The listing builds one solid part. Answer for the finished solid, in the listing's coordinates (mm). Face numbers are marked on the shaded views. A direction names the side the tool comes from. Coordinates: 2 decimals unless noted, no trailing zeros. Loops run counter-clockwise (first coordinate to the right, second up) from the corner with the lowest first, then second, coordinate; pieces in that order, holes last. Notation, with made-up numbers: (7, 74.5) - (15, 74.5) arc R23 ccw to (15, 103.5) - close; hole circle Ø8 at (32, 31.25). An arc over 180 degrees is marked (long way). Put each result on its own line as item: value.
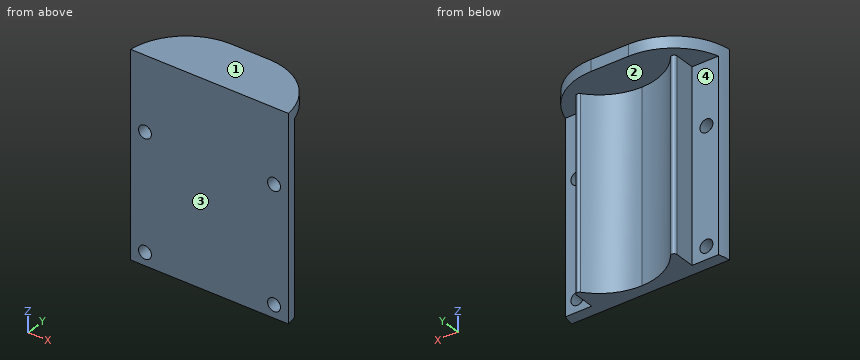
```python
from build123d import *

# Parameters (mm, degrees)
SKETCH1_W            = 55
SKETCH1_H            = 70
BOSS_EXTRUDE1_DEPTH  = 4
M4_CLEARANCE_HOLE1_D = 4.5
BOSS_EXTRUDE2_DEPTH  = 70
SKETCH5_W            = 55
SKETCH5_H            = 4
BOSS_EXTRUDE3_DEPTH  = 15
FILLET1_R            = 1
FILLET2_START        = -36
FILLET2_DEPTH        = 71


with BuildPart() as part:
    # Sketch1 → Boss-Extrude1 (new body)
    with BuildSketch(Plane(origin=(0, 0, 0), x_dir=(1, 0, 0), z_dir=(0, 1, 0))):
        Rectangle(SKETCH1_W, SKETCH1_H)
    extrude(amount=BOSS_EXTRUDE1_DEPTH)

    # M4 Clearance Hole1 (through all)
    with Locations(Plane(origin=(0, 4, 0), x_dir=(1, 0, 0), z_dir=(0, 1, 0))):
        with Locations((-22.5, 30.536735359), (22.5, 30.536735359), (-22.5, -9.463264641), (22.5, -9.463264641)):
            Hole(M4_CLEARANCE_HOLE1_D / 2)

    # Sketch4 → Boss-Extrude2 (add, through all)
    with BuildSketch(Plane(origin=(0, 0, -35), x_dir=(-1, 0, 0), z_dir=(0, 0, -1))):
        with BuildLine():
            Line((-17.5, 14.317541634), (-17.5, 4))
            Line((-17.5, 4), (0, 4))
            ThreePointArc((0, 4), (-10.157530032, 6.771402156), (-17.5, 14.317541634))
        make_face()
        with BuildLine():
            ThreePointArc((17.5, 14.317541634), (10.157530032, 6.771402156), (0, 4))
            Line((0, 4), (17.5, 4))
            Line((17.5, 4), (17.5, 14.317541634))
        make_face()
    extrude(amount=-BOSS_EXTRUDE2_DEPTH)

    # Sketch5 → Boss-Extrude3 (add)
    with BuildSketch(Plane(origin=(0, 4, 0), x_dir=(1, 0, 0), z_dir=(0, 1, 0))):
        with Locations((0, -33)):
            Rectangle(SKETCH5_W, SKETCH5_H)
    extrude(amount=BOSS_EXTRUDE3_DEPTH)

    # Fillet1
    fillet1_edges = [part.edges().sort_by_distance(p)[0] for p in [
        (-17.5, 14.317541634, -2),
        (17.5, 14.317541634, -2),
    ]]
    fillet(fillet1_edges, radius=FILLET1_R)

    # Fillet2: read off the stored shape, not the designer's step
    # Fillet2 outline → Fillet2 (cut)
    with BuildSketch(Plane.XY.offset(FILLET2_START)):
        with BuildLine():
            ThreePointArc((-27.5, 0), (-20.719901931, 13.540270268), (-6.59545504, 19))
            Line((-6.59545504, 19), (-27.5, 19))
            Line((-27.5, 19), (-27.5, 0))
        make_face()
        with BuildLine():
            ThreePointArc((6.59545504, 19), (20.719901931, 13.540270268), (27.5, 0))
            Line((27.5, 0), (27.5, 19))
            Line((27.5, 19), (6.59545504, 19))
        make_face()
    extrude(amount=FILLET2_DEPTH, mode=Mode.SUBTRACT)


solid = part.part
```
1) The part is cut by section C-C (y = 16.25). Give the vertices of the cut face in (x, z), and give its area (3 significant figures).
Found:
outline: (-16.98, 31) - (16.98, 31) - (16.98, 35) - (-16.98, 35) - close
area: 136 mm^2
2) Each of these flat-tipped pins is pushed along its axis until it touches: pin 1 (12 mm diameter, centred on x = 4, z = -14, fed in from +Y); pin 2 (7 mm diameter, centred on x = -22.5, z = 9.46, fed in from +Y); pin 3 (1.5 mm diameter, centred on x = 16.5, z = -7.5, fed in from +Y). Where does it stop, or does it pass through?
Found:
pin 1: stops at y = 6.68
pin 2: stops at y = 4
pin 3: stops at y = 12.01
3) For the marked faces 3 and 4, determine the directions among +Z, -Z, +X, -X, +Y, -Y from which every point of the face is accessible in a straight line to the end or side of a thin tool.
Found:
face 3: +Z, -Z, +X, -X, -Y
face 4: -Z, -X, +Y
4) The part is cut by section D-D (x = -8.5). Give the vertices of the cut face in (y, z).
Found:
outline: (0, -35) - (5.9, -35) - (5.9, 31) - (18.91, 31) - (18.91, 35) - (0, 35) - close
5) Straight lines are drawn through the part: L1, parallel to Z at x = 22.5, y = 1.65; L2, parallel to Y at x = -21, z = -23; L3, parallel to X at y = 11.5, z = 2. For each, find the intervals that lie inside material, in ascending order. Write a range as [from, to].
Found:
L1: z = [-35, -32.79], [-28.29, 7.21], [11.71, 35]
L2: y = [0, 4]
L3: x = [-17.37, -15.61], [15.61, 17.37]
6) The part is cut by section B-B (z = -6.5). Give the vertices of the cut face in (x, y).
Found:
outline: (-27.5, 0) - (27.5, 0) arc R21 ccw to (26.72, 4) - (17.5, 4) - (17.5, 11.01) arc R1 ccw to (15.71, 11.63) arc R20 cw to (-15.71, 11.63) arc R1 ccw to (-17.5, 11.01) - (-17.5, 4) - (-26.72, 4) arc R21 ccw to start
7) The part is cut by section A-A (x = -23). Give the vertices of the cut face in (y, z), and give its area (3 significant figures).
Found:
outline: (0, -35) - (4, -35) - (4, -32.73) - (0, -32.73) - close; (0, -28.34) - (4, -28.34) - (4, 7.27) - (0, 7.27) - close; (0, 11.66) - (4, 11.66) - (4, 31) - (11.11, 31) - (11.11, 35) - (0, 35) - close
area: 273 mm^2
8) For a pull along X with two mould halves and no side action, classify the marked faces 1 and 2 as pulls with the +X half, pulls with the -X half, needs draft (parallel to the pull), parting line crosses it, or undercut.
Found:
face 1: needs draft
face 2: undercut
